Build history of the part. All positions in model axes, mm. A direction names the side the tool comes from. Round coordinates to 2 decimals unless told otherwise and drop trailing zeros. Loops run counter-clockwise (first coordinate to the right, second up) from the corner with the lowest first, then second, coordinate; pieces in that order, holes last. Notation, with made-up numbers: M -21.5,36.5 L 14.5,36.5 A11 ccw 14.5,45.5 Z; hole C -27,6 d6. An arc over 180 degrees is marked long. One line per item, written item: value.
```python
from build123d import *

# Parameters (mm, degrees)
SKETCH1_R           = 19
BOSS_EXTRUDE1_DEPTH = 1
SKETCH2_R           = 18
SKETCH2_R_2         = 16
BOSS_EXTRUDE2_DEPTH = 10
SKETCH3_W           = 3
SKETCH3_H           = 2
SKETCH3_W_2         = 2
SKETCH3_H_2         = 3
CUT_EXTRUDE1_DEPTH  = 10


with BuildPart() as part:
    # Sketch1 → Boss-Extrude1 (new body)
    with BuildSketch(Plane(origin=(0, 0, 0), x_dir=(0, 1, 0), z_dir=(0, 0, 1))):
        with Locations(Location((0, 0, 0), (0, 0, 270))):
            Circle(SKETCH1_R)
    extrude(amount=BOSS_EXTRUDE1_DEPTH)

    # Sketch2 → Boss-Extrude2 (add)
    with BuildSketch(Plane.XY.offset(1)):
        Circle(SKETCH2_R)
        Circle(SKETCH2_R_2, mode=Mode.SUBTRACT)
    extrude(amount=BOSS_EXTRUDE2_DEPTH)

    # Sketch3 → Cut-Extrude1 (cut)
    with BuildSketch(Plane.XY.offset(11)):
        with Locations((17, 0)):
            Rectangle(SKETCH3_W, SKETCH3_H)
        with Locations((0, 17)):
            Rectangle(SKETCH3_W_2, SKETCH3_H_2)
        with Locations((0, -17)):
            Rectangle(SKETCH3_W_2, SKETCH3_H_2)
        with Locations((-17, 0)):
            Rectangle(SKETCH3_W, SKETCH3_H)
    extrude(amount=-CUT_EXTRUDE1_DEPTH, mode=Mode.SUBTRACT)


solid = part.part
```
Item 1: Pull direction X, two halves, no side cores. Call faces 1 (the face through (-11.428, -11.199, 5.93)), 2 (the face through (-17, -1, 6)), 3 (the face through (12.857, 12.597, 5.93)), 4 (the face through (-12.857, -12.597, 5.93)): pulls with the +X half, pulls with the -X half, needs draft (parallel to the pull), parting line crosses it, or undercut.
Check values:
face 1: undercut
face 2: needs draft
face 3: pulls with the +X half
face 4: pulls with the -X half
Item 2: Slice it at C-C, the plane x = -10. Give the cut face in (y, z), and give its area (3 significant figures).
Check values:
outline: M -16.16,0 L 16.16,0 L 16.16,1 L 14.97,1 L 14.97,11 L 12.49,11 L 12.49,1 L -12.49,1 L -12.49,11 L -14.97,11 L -14.97,1 L -16.16,1 Z
area: 81.8 mm2
Item 3: Slice it at D-D, the plane x = 0. Give the cut face in (y, z), and give its area (3 significant figures).
Check values:
outline: M -19,0 L 19,0 L 19,1 L -19,1 Z
area: 38.0 mm2
Item 4: Drop flat-ended pins along their axis: P1, Ø1.6, axis at x = -16.5, z = 6, coming from the -Y side; P2, Ø2, axis at x = -13, y = -5.5, coming from the +Z side; P3, Ø1.6, axis at x = 17, z = 5, coming from the +Y side. Give the stop position or say it passes through.
Check values:
P1: stops at y = -8.8
P2: stops at z = 1
P3: stops at y = 7.85
Item 5: Wall check: line 1 along X through (y, z) = (10, 8); line 2 along X through (y, z) = (16.5, 2); line 3 along Z through (x, y) = (1, 7.5). Give the ranges that are in metal, low to high.
Check values:
line 1: x = -14.97 to -12.49, 12.49 to 14.97
line 2: x = -7.19 to -1, 1 to 7.19
line 3: z = 0 to 1
Item 6: Which spindle directions (+Z, -Z, +X, -X, +Y, -Y) get a long thin tool onto all of the face, cutting with end or side? Do faces 5 (the face through (-12.597, 12.857, 5.93)), 6 (the face through (17, -1, 6)), 7 (the face through (11.199, -11.428, 5.93)), 8 (the face through (-1, -17, 6)). Say none if no direction does.
Check values:
face 5: +Z, -X, +Y
face 6: +Z, +X, -X
face 7: +Z
face 8: +Z, +Y, -Y
Item 7: Slice it at B-B, the plane y = -12. Give the cut face in (x, z).
Check values:
outline: M -14.73,0 L 14.73,0 L 14.73,1 L 13.42,1 L 13.42,11 L 10.58,11 L 10.58,1 L -10.58,1 L -10.58,11 L -13.42,11 L -13.42,1 L -14.73,1 Z
Item 8: Slice it at A-A, the plane z = 4.5. Give the cut face in (x, y), and give its area (3 significant figures).
Check values:
outline: M -17.97,-1 A18 ccw -1,-17.97 L -1,-15.97 A16 cw -15.97,-1 Z; M -17.97,1 L -15.97,1 A16 cw -1,15.97 L -1,17.97 A18 ccw Z; M 1,-17.97 A18 ccw 17.97,-1 L 15.97,-1 A16 cw 1,-15.97 Z; M 1,15.97 A16 cw 15.97,1 L 17.97,1 A18 ccw 1,17.97 Z
area: 198 mm2
